Geometry: final body of the model. Coordinates: model frame, mm. Round coordinates to 2 decimals unless told otherwise and drop trailing zeros. Loops run counter-clockwise (first coordinate to the right, second up) from the corner with the lowest first, then second, coordinate; pieces in that order, holes last. Notation, with made-up numbers: (43, 36.25) - (49, 36.25) arc R20 ccw to (49, 46.25) - close; hole circle Ø3 at (49, 2.25). An arc over 180 degrees is marked (long way). Answer as a JSON object with one key per item and string values. Group by question number.
Item 1: Draft query along X for faces 1 (the face through (3, -3, 10)), 2 (the face through (0, 0, 0)), 3 (the face through (56.228, 8.057, -12.637)). Return one class per face: released by +X, released by -X, zero draft, split by the parting line, or undercut.
Item 2: Line query: line 1 (X direction, y = 0.5, z = 13); line 2 (X direction, y = -2, z = -11.5); line 3 (Z direction, x = 73, y = 12.5). Output: solid intervals per line, ascending.
Item 3: Section A-A (z = 0). Return the cut outline in (x, y), plus the area to 3 significant figures.
Item 4: First-contact query: pin 1 (12 mm diameter, centred on x = 24.5, z = 8.5, fed in from -Y); pin 2 (8 mm diameter, centred on x = 50, z = 6, fed in from -Y); pin 3 (1 mm diameter, centred on x = 37.5, y = -4.5, fed in from +Z). Flat tips, straight axial feed; report the tip coordinate or a pass-through.
Item 5: Section D-D (x = 64.5). Return the cut outline in (y, z).
Item 6: Section C-C (x = 18.5). Return the cut outline in (y, z).
```python
from build123d import *


with BuildPart() as part:
    # Sketch1 → Revolve1 (revolve)
    with BuildSketch(Plane.XY):
        with BuildLine():
            Line((0, 15), (0, 0))
            Line((0, 0), (100, 0))
            ThreePointArc((100, 0), (95.828314101, 10.380154803), (85.633651502, 14.986610216))
            Line((85.633651502, 14.986610216), (27.634324528, 14.986610216))
            ThreePointArc((27.634324528, 14.986610216), (24.337461443, 13.403793666), (23, 10))
            Line((23, 10), (3, 10))
            Line((3, 10), (3, 15))
            ThreePointArc((3, 15), (1.5, 16.5), (0, 15))
        make_face()
    revolve(axis=Axis((100, 0, 0), (-1, 0, 0)))


solid = part.part
```
Values:
{
 "1": {"face 1": "undercut", "face 2": "released by -X", "face 3": "zero draft"},
 "2": {"line 1": "x = 0 to 3, 24.01 to 92.47", "line 2": "x = 0 to 3, 23.29 to 94.42", "line 3": "z = -8.27 to 8.27"},
 "3": {"outline": "(0, -15) arc R1.5 ccw to (3, -15) - (3, -10) - (23, -10) arc R5 ccw to (27.63, -14.99) - (85.63, -14.99) arc R15 ccw to (85.63, 14.99) - (27.63, 14.99) arc R5 ccw to (23, 10) - (3, 10) - (3, 15) arc R1.5 ccw to (0, 15) - close", "area": "2,700 mm^2"},
 "4": {"pin 1": "stops at y = -14.61", "pin 2": "stops at y = -14.85", "pin 3": "stops at z = 14.44"},
 "5": {"outline": "circle Ø29.97 at (0, 0)"},
 "6": {"outline": "circle Ø20 at (0, 0)"}
}
